Part model, mm, in its own coordinate system. A direction names the side the tool comes from. Round coordinates to 2 decimals unless told otherwise and drop trailing zeros. Order: outer loops, then holes, each group sorted by start corner. A loop starts at its lowest first (then second) coordinate and runs counter-clockwise, first axis right, second up. Notation, with made-up numbers: (66, 17.25) - (100, 17.25) arc R25 ccw to (100, 35.25) - close; hole circle Ø11 at (-17, -9). An arc over 180 degrees is marked (long way). Answer as a JSON object with one key per item and string values.
```python
from build123d import *

# Parameters (mm, degrees)
BOSS_EXTRUDE1_DEPTH      = 400
SKETCH2_R                = 2.1
CUT_EXTRUDE3_DEPTH       = 10
SKETCH3_W                = 158.039132068
SKETCH3_H                = 497.98789011
CUT_EXTRUDE4_DEPTH       = 2
SKETCH4_W                = 4.8
SKETCH4_H                = 400
BOSS_EXTRUDE2_DEPTH      = 8
SKETCH5_R                = 1.2
CUT_EXTRUDE9_DEPTH       = 406.158043237
SKETCH9_R                = 1.225
CUT_EXTRUDE10_DEPTH      = 406.931077894
SKETCH10_W               = 4.8
SKETCH10_H               = 400
CUT_EXTRUDE11_DEPTH      = 5
BOSS_EXTRUDE3_START      = -15
SKETCH12_R               = 2.1
BOSS_EXTRUDE3_DEPTH      = 15
SKETCH13_W               = 6.18
SKETCH13_H               = 37.25
BOSS_EXTRUDE5_DEPTH      = 10
BOSS_EXTRUDE6_DEPTH      = 6.18
SKETCH15_R               = 1.05
CUT_EXTRUDE12_DEPTH      = 10
FILLET1_R                = 2
SKETCH16_W               = 4.8
SKETCH16_H               = 400
CUT_EXTRUDE13_DEPTH      = 2.5
CUT_EXTRUDE14_REACH      = 404.247
SKETCH17_R               = 1.16
CUT_EXTRUDE16_DEPTH      = 406.158043237
CUT_EXTRUDE16_DEPTH_BACK = 406.158043237
SKETCH18_R               = 1.225
CUT_EXTRUDE17_DEPTH      = 406.158043237
CUT_EXTRUDE17_DEPTH_BACK = 406.158043237
SKETCH20_R               = 1.225
SKETCH22_W               = 3
SKETCH22_H               = 15
CUT_EXTRUDE18_DEPTH      = 406.931077894
FILLET2_R                = 2
FILLET3_R                = 2
SKETCH24_W               = 3
SKETCH24_H               = 200
SKETCH24_W_2             = 2
CUT_EXTRUDE20_DEPTH      = 406.931077894


with BuildPart() as part:
    # Sketch1 → Boss-Extrude1 (new body)
    with BuildSketch(Plane.XY):
        Polygon((0, 0), (0, 25), (5, 25), (5, 5), (60.2, 5), (60.2, 25), (65.2, 25), (65.2, 0), align=None)
    extrude(amount=BOSS_EXTRUDE1_DEPTH)

    # Sketch2 → Cut-Extrude3 (cut)
    with BuildSketch(Plane(origin=(0, 5, 0), x_dir=(1, 0, 0), z_dir=(0, 1, 0))):
        with Locations(Location((32.6, -67.17, 0), (0, 0, 270))):
            Circle(SKETCH2_R)
        with Locations(Location((32.6, -96.92, 0), (0, 0, 270))):
            Circle(SKETCH2_R)
    extrude(amount=-CUT_EXTRUDE3_DEPTH, mode=Mode.SUBTRACT)

    # Sketch3 → Cut-Extrude4 (cut)
    with BuildSketch(Plane(origin=(0, 25, 0), x_dir=(1, 0, 0), z_dir=(0, 1, 0))):
        with Locations((44.123686713, -201.646240959)):
            Rectangle(SKETCH3_W, SKETCH3_H)
    extrude(amount=-CUT_EXTRUDE4_DEPTH, mode=Mode.SUBTRACT)

    # Sketch4 → Boss-Extrude2 (add)
    with BuildSketch(Plane(origin=(0, 5, 0), x_dir=(1, 0, 0), z_dir=(0, 1, 0))):
        with Locations((7.4, -200)):
            Rectangle(SKETCH4_W, SKETCH4_H)
        with Locations((57.8, -200)):
            Rectangle(SKETCH4_W, SKETCH4_H)
    extrude(amount=BOSS_EXTRUDE2_DEPTH)

    # Sketch5 → Cut-Extrude9 (cut, through all)
    with BuildSketch(Plane(origin=(5, 0, 0), x_dir=(0, 0, -1), z_dir=(1, 0, 0))):
        with Locations(Location((-395, 16.5, 0), (0, 0, 90))):
            Circle(SKETCH5_R)
        with Locations(Location((-390, 16.5, 0), (0, 0, 90))):
            Circle(SKETCH5_R)
        with Locations(Location((-10, 16.5, 0), (0, 0, 90))):
            Circle(SKETCH5_R)
        with Locations(Location((-5, 16.5, 0), (0, 0, 90))):
            Circle(SKETCH5_R)
    extrude(amount=-CUT_EXTRUDE9_DEPTH, mode=Mode.SUBTRACT)

    # Sketch9 → Cut-Extrude10 (cut, through all)
    with BuildSketch(Plane.ZY):
        with Locations((5, 16.5)):
            Circle(SKETCH9_R)
        with Locations((10, 16.5)):
            Circle(SKETCH9_R)
        with Locations((390, 16.5)):
            Circle(SKETCH9_R)
        with Locations((395, 16.5)):
            Circle(SKETCH9_R)
    extrude(amount=-CUT_EXTRUDE10_DEPTH, mode=Mode.SUBTRACT)

    # Sketch10 → Cut-Extrude11 (cut)
    with BuildSketch(Plane(origin=(0, 13, 0), x_dir=(1, 0, 0), z_dir=(0, 1, 0))):
        with Locations((7.4, -200)):
            Rectangle(SKETCH10_W, SKETCH10_H)
        with Locations((57.8, -200)):
            Rectangle(SKETCH10_W, SKETCH10_H)
    extrude(amount=-CUT_EXTRUDE11_DEPTH, mode=Mode.SUBTRACT)

    # Sketch12 → Boss-Extrude3 (add)
    with BuildSketch(Plane.XZ.offset(BOSS_EXTRUDE3_START)):
        with Locations(Location((32.6, 96.92, 0), (0, 0, 270))):
            Circle(SKETCH12_R)
        with Locations(Location((32.6, 67.17, 0), (0, 0, 270))):
            Circle(SKETCH12_R)
    extrude(amount=BOSS_EXTRUDE3_DEPTH)

    # Sketch13 → Boss-Extrude5 (add)
    with BuildSketch(Plane(origin=(0, 5, 0), x_dir=(1, 0, 0), z_dir=(0, 1, 0))):
        with Locations((32.6, -82.045)):
            Rectangle(SKETCH13_W, SKETCH13_H)
    extrude(amount=BOSS_EXTRUDE5_DEPTH)

    # Sketch14 → Boss-Extrude6 (add)
    with BuildSketch(Plane.ZY.offset(-29.51)):
        Polygon((70.92, 15), (75.32, 19.4), (88.77, 19.4), (93.17, 15), align=None)
    extrude(amount=-BOSS_EXTRUDE6_DEPTH)

    # Sketch15 → Cut-Extrude12 (cut)
    with BuildSketch(Plane.ZY.offset(-29.51)):
        with Locations((78.87, 16)):
            Circle(SKETCH15_R)
        with Locations((85.22, 16)):
            Circle(SKETCH15_R)
    extrude(amount=-CUT_EXTRUDE12_DEPTH, mode=Mode.SUBTRACT)

    # Fillet1
    fillet1_edges = [part.edges().sort_by_distance(p)[0] for p in [
        (29.51, 5, 82.045),
        (29.51, 10, 63.42),
        (32.6, 5, 100.67),
        (29.51, 10, 100.67),
        (35.69, 5, 82.045),
        (35.69, 10, 100.67),
        (32.6, 5, 63.42),
        (35.69, 10, 63.42),
    ]]
    fillet(fillet1_edges, radius=FILLET1_R)

    # Sketch16 → Cut-Extrude13 (cut)
    with BuildSketch(Plane(origin=(0, 8, 0), x_dir=(1, 0, 0), z_dir=(0, 1, 0))):
        with Locations((7.4, -200)):
            Rectangle(SKETCH16_W, SKETCH16_H)
        with Locations((57.8, -200)):
            Rectangle(SKETCH16_W, SKETCH16_H)
    extrude(amount=-CUT_EXTRUDE13_DEPTH, mode=Mode.SUBTRACT)

    # Sketch17 → Cut-Extrude14 (cut, up to next)
    with BuildSketch(Plane.ZY.offset(-29.51), mode=Mode.PRIVATE) as cut_extrude14_sk1:
        with Locations((78.87, 16)):
            Circle(SKETCH17_R)
    cut_extrude14_tool1 = extrude(cut_extrude14_sk1.sketch, amount=-CUT_EXTRUDE14_REACH, mode=Mode.PRIVATE) & part.part
    # Sketch17 → Cut-Extrude14 (cut, up to next)
    with BuildSketch(Plane.ZY.offset(-29.51), mode=Mode.PRIVATE) as cut_extrude14_sk2:
        with Locations((85.22, 16)):
            Circle(SKETCH17_R)
    cut_extrude14_tool2 = extrude(cut_extrude14_sk2.sketch, amount=-CUT_EXTRUDE14_REACH, mode=Mode.PRIVATE) & part.part
    add(cut_extrude14_tool1.solids().sort_by_distance((29.51, 16, 78.87))[0], mode=Mode.SUBTRACT)
    add(cut_extrude14_tool2.solids().sort_by_distance((29.51, 16, 85.22))[0], mode=Mode.SUBTRACT)

    # Sketch18 → Cut-Extrude16 (cut, two sides: drawn at the far end of the back side and taken through both)
    with BuildSketch(Plane.ZY.offset(-60.2).offset(-CUT_EXTRUDE16_DEPTH_BACK)):
        with Locations((170, 16.5)):
            Circle(SKETCH18_R)
    extrude(amount=CUT_EXTRUDE16_DEPTH + CUT_EXTRUDE16_DEPTH_BACK, mode=Mode.SUBTRACT)

    # Sketch20 → Cut-Extrude17 (cut, two sides: drawn at the far end of the back side and taken through both)
    with BuildSketch(Plane.ZY.offset(-60.2).offset(-CUT_EXTRUDE17_DEPTH_BACK)):
        with Locations((230, 16.5)):
            Circle(SKETCH20_R)
    extrude(amount=CUT_EXTRUDE17_DEPTH + CUT_EXTRUDE17_DEPTH_BACK, mode=Mode.SUBTRACT)

    # Sketch22 → Cut-Extrude18 (cut, through all)
    with BuildSketch(Plane(origin=(0, 0, 0), x_dir=(-1, 0, 0), z_dir=(0, 0, -1))):
        with Locations((-63.7, 15.5)):
            Rectangle(SKETCH22_W, SKETCH22_H)
        with Locations((-1.5, 15.5)):
            Rectangle(SKETCH22_W, SKETCH22_H)
    extrude(amount=-CUT_EXTRUDE18_DEPTH, mode=Mode.SUBTRACT)

    # Fillet2
    fillet2_edges = [part.edges().sort_by_distance(p)[0] for p in [
        (62.2, 8, 200),
    ]]
    fillet(fillet2_edges, radius=FILLET2_R)

    # Fillet3
    fillet3_edges = [part.edges().sort_by_distance(p)[0] for p in [
        (3, 8, 200),
    ]]
    fillet(fillet3_edges, radius=FILLET3_R)

    # Sketch24 → Cut-Extrude20 (cut, through all)
    with BuildSketch(Plane(origin=(0, 23, 0), x_dir=(1, 0, 0), z_dir=(0, 1, 0))):
        Polygon((22.6, -200), (0, -200), (0, -400), (60.2, -400), (60.2, -200), (42.6, -200), (42.6, -220), (22.6, -220), align=None)
        with Locations((63.7, -300)):
            Rectangle(SKETCH24_W, SKETCH24_H)
        with Locations((61.2, -300)):
            Rectangle(SKETCH24_W_2, SKETCH24_H)
    extrude(amount=-CUT_EXTRUDE20_DEPTH, mode=Mode.SUBTRACT)


solid = part.part
```
Item 1: Cut at A-A (z = 51.5). Write the cut outline in (x, y).
Taken from the geometry:
{"outline": "(0, 0) - (65.2, 0) - (65.2, 8) - (64.2, 8) arc R2 cw to (62.2, 10) - (62.2, 23) - (60.2, 23) - (60.2, 5.5) - (55.4, 5.5) - (55.4, 5) - (9.8, 5) - (9.8, 5.5) - (5, 5.5) - (5, 23) - (3, 23) - (3, 10) arc R2 cw to (1, 8) - (0, 8) - close"}
Item 2: Tool access for faces 1 (the flat face through (32.56, 17.17, 73.09)), 2 (the flat face through (9.7, 4.7, 200)), 3 (the flat face through (33, 15, 97)), 4 (the flat face through (5, 14, 101)), 5 (the flat face through (42.6, 3, 210)): list every direction of +Z, -Z, +X, -X, +Y, -Y with a clear straight run to the whole face (end or side of a thin tool).
Taken from the geometry:
{"face 1": "-Z, +Y", "face 2": "+Z, -X, +Y, -Y", "face 3": "+Z, +Y", "face 4": "+Z, -Z, +Y", "face 5": "+Z, +X, +Y, -Y"}
Item 3: Probe L1, parallel to X at y = 17, z = 88.5; L2, parallel to X at y = 11.5, z = 19; L3, parallel to Y at x = 4.35, z = 170 (3 decimals). List the from-to ranges inside material, lowest first. Write a range as from..to.
Taken from the geometry:
{"L1": "3..5, 29.51..35.69, 60.2..62.2", "L2": "3..5, 60.2..62.2", "L3": "0..15.275, 17.725..23"}
Item 4: Drop flat-ended pins along their axis: P1, Ø12, axis at x = 52.5, y = 13.5, coming from the -Z side; P2, Ø5.5, axis at y = 1.5, z = 208, coming from the +X side; P3, Ø1.5, axis at x = 25, z = 183, coming from the +Y side; P4, Ø5, axis at x = 32.5, z = 67.5, coming from the +Y side. Give the stop position or say it passes through.
Taken from the geometry:
{"P1": "through", "P2": "x = 42.6", "P3": "y = 5", "P4": "y = 15"}
Item 5: Cut at B-B (z = 203.5). Write the cut outline in (x, y).
Taken from the geometry:
{"outline": "(22.6, 0) - (42.6, 0) - (42.6, 5) - (22.6, 5) - close"}
Item 6: Two-plate mould, pull along X, no slides. Class faces 6 (the flat face through (58, 5.5, 99)), 7 (the flat face through (33, 3, 220)), 8 (the flat face through (62.2, 16, 99)), 9 (the flat face through (33, 19.4, 82)): pulls with the +X half, pulls with the -X half, needs draft (parallel to the pull), parting line crosses it, or undercut.
Taken from the geometry:
{"face 6": "undercut", "face 7": "needs draft", "face 8": "pulls with the +X half", "face 9": "undercut"}
